Build history of the part. All positions in model axes, mm. Face numbers are marked on the shaded views. Round coordinates to 2 decimals unless told otherwise and drop trailing zeros. Write each loop counter-clockwise with the first axis right and the second up, starting at its lowest first coordinate (ties: lowest second). Pieces come first, ordered by that corner, then holes. Notation, with made-up numbers: (-36, 43) - (-18, 43) arc R12 ccw to (-18, 58) - close; hole circle Ø2 at (44.25, -25). An arc over 180 degrees is marked (long way). One line per question, with ' | ' between items.
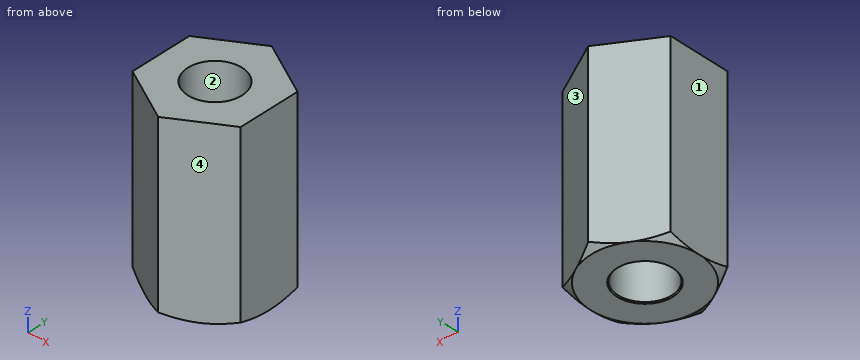
from build123d import *

# Parameters (mm, degrees)
EXTRUDE1_DEPTH      = 5
EXTRUDE1_DEPTH_BACK = 5
SKETCH1_R           = 1.5
SKETCH8_OUTSIDE_W   = 52.282
SKETCH8_OUTSIDE_H   = 53.21
SKETCH8_OUTSIDE_R   = 3
EXTRUDE4_DEPTH      = 12
EXTRUDE4_DRAFT      = -60


with BuildPart() as part:
    # Sketch1 → Extrude1 (new, two sides: drawn at the far end of the back side and taken through both)
    with BuildSketch(Plane.XY.offset(-EXTRUDE1_DEPTH_BACK)):
        Polygon((0, 3.464101615), (-3, 1.732050808), (-3, -1.732050808), (0, -3.464101615), (3, -1.732050808), (3, 1.732050808), align=None)
        Circle(SKETCH1_R, mode=Mode.SUBTRACT)
    extrude(amount=EXTRUDE1_DEPTH + EXTRUDE1_DEPTH_BACK)

    # Extrude3 cone 1 section (through the dimple's axis) → Extrude3 (revolve, cut)
    with BuildSketch(Plane(origin=(0, 0, -5), x_dir=(0, 1, 0), z_dir=(1, 0, 0))):
        Polygon((0, 0), (1.5508, 0), (0, 1.663029396), align=None)
    revolve(axis=Axis((0, 0, -5), (0, 0, 1)), mode=Mode.SUBTRACT)


with BuildPart() as extrude4_tool:
    # Sketch8 outside → Extrude4 (with draft: the straight prism first)
    with BuildSketch(Plane(origin=(0, 0, -5), x_dir=(-1, 0, 0), z_dir=(0, 0, -1))):
        Rectangle(SKETCH8_OUTSIDE_W, SKETCH8_OUTSIDE_H)
        Circle(SKETCH8_OUTSIDE_R, mode=Mode.SUBTRACT)
    extrude(amount=-EXTRUDE4_DEPTH)
    # Extrude4: the draft: its side faces are tilted about the plane it starts from
    extrude4_sides = [extrude4_tool.faces().sort_by_distance(p)[0] for p in [
        (0, -26.605, 1),
        (-26.141, 0, 1),
        (0, 26.605, 1),
        (26.141, 0, 1),
        (3, 0, 1),
    ]]
    draft(extrude4_sides, Plane(origin=(0, 0, -5), x_dir=(-1, 0, 0), z_dir=(0, 0, -1)), EXTRUDE4_DRAFT)


with BuildPart() as part_1:
    add(part.part)

    # Extrude4: cut by extrude4_tool
    add(extrude4_tool.part, mode=Mode.SUBTRACT)


solid = part_1.part
Q1. Drop a flat-ended pin along its axis: pin 1 (1.5 mm diameter, centred on x = 1.5, z = 2, fed in from -Y). Give the stop position or say it passes through.
Found:
pin 1: y = -3.03
Q2. Drill centre lines: L1, parallel to X at y = 0, z = 1; L2, parallel to Y at x = 0.75, z = 3.5; L3, parallel to Y at x = 0.25, z = -2.25. Where is each one in solid material? Low to high. Write a range as from..to.
Found:
L1: -3..-1.5, 1.5..3 | L2: -3.03..-1.3, 1.3..3.03 | L3: -3.32..-1.48, 1.48..3.32
Q3. Saw through at A-A, the plane z = -3.75. List the corners of the cut face in (x, y).
Found:
outline: (-3, -1.73) - (0, -3.46) - (3, -1.73) - (3, 1.73) - (0, 3.46) - (-3, 1.73) - close; hole circle Ø3 at (0, 0)
Q4. Pull direction Y, two halves, no side cores. Call the marked faces 1, 2, 3 and 4: +Y half, -Y half, draft (parallel to the pull), parting line (faces both ways), or undercut.
Found:
face 1: draft | face 2: undercut | face 3: +Y half | face 4: -Y half
